Build history of the part. All positions in model axes, mm. A direction names the side the tool comes from. Round coordinates to 2 decimals unless told otherwise and drop trailing zeros. Write each loop counter-clockwise with the first axis right and the second up, starting at its lowest first coordinate (ties: lowest second). Pieces come first, ordered by that corner, then holes.
Autodesk Inventor part; units mm, degrees
ref_plane "YZ Plane" through (0, 0, 0) normal (1, 0, 0) x (0, 1, 0)
ref_plane "XZ Plane" through (0, 0, 0) normal (0, 1, 0) x (-1, 0, 0)
ref_plane "XY Plane" through (0, 0, 0) normal (0, 0, 1) x (1, 0, 0)
sketch "Sketch1" plane through (0, 0, 0) normal (0, 0, 1) x (1, 0, 0)
  line L0 (-20, 75) -> (20, 75)
  line L1 (20, 75) -> (20, -75)
  line L2 (20, -75) -> (-20, -75)
  line L3 (-20, -75) -> (-20, 75)
  line L4 (-20, 75) -> (20, -75) construction
  line L5 (20, 75) -> (-20, -75) construction
  point P0 (0, 0)
  point P1 (0, 0)
  dimension "d0" = 40
  dimension "d1" = 150
extrude "Plate1" add sketch "Sketch1" along normal blind 2
sketch "Sketch2" plane through (-20, -75, 2) normal (-1, 0, 0) x (0, -1, 0)
  line L0 (-150, 0) -> (0, 0)
  line L1 (0, 0) -> (0, 33)
  line L2 (0, 33) -> (-150, 33)
  line L3 (-150, 33) -> (-150, 0)
edge flange "Flange1" height 35 angle 90 thickness 2 bend radius 2 thickness toward (-1, 0, 0) relief tear relief width 2 relief depth 1 corner gap 2 corner form 0 edges at (-20, 0, 2) (20, 0, 2) wall of the first edge with corners at (-20, 75, 2) (-20, -75, 2) (-20, -75, 35) (-20, 75, 35)
bend "Bend1"
corner "Corner1"
sketch "Sketch3" plane through (0, 0, 0) normal (1, 0, 0) x (0, 1, 0)
  line L0 (-75, 4) -> (75, 4)
  line L1 (75, 35) -> (75, 4)
  line L2 (-75, 35) -> (75, 35)
  line L3 (-75, 4) -> (-75, 35)
  circle A0 centre (-55, 22) radius 2.5
  line L4 (-55, 22.75) -> (-55, 21.25) construction
  line L5 (-57.5, 22.75) -> (-57.5, 21.25)
  line L6 (-52.5, 21.25) -> (-52.5, 22.75)
  arc A1 (-52.5, 22.75) -> (-57.5, 22.75) centre (-55, 22.75) ccw
  arc A2 (-57.5, 21.25) -> (-52.5, 21.25) centre (-55, 21.25) ccw
  point P0 (0, 0)
  point P1 (-52.5, 22)
  point P2 (-57.5, 22)
  dimension "d13" = 5
  dimension "d14" = 13
  dimension "d15" = 20
  dimension "d29" = 1.5
extrude "Extrusion1" cut sketch "Sketch3" along normal through all both and the other way through all contours A0 | L6 A2 L5 A0 | A0 L5 A1 L6
pattern_linear "Rectangular Pattern2" count 2 spacing 100 along (0, 1, 0) of "Extrusion1"
fillet "Fillet1" radius 2 4 edges at (-21, -75, 35) (21, -75, 35) (-21, 75, 35) (21, 75, 35)
equation "\"d2\" = Thickness"
equation "\"d3\" = BendReliefWidth"
equation "\"d4\" = BendReliefDepth"
equation "\"d5\" = MinimumRemnant"
equation "\"d6\" = TransitionRadius"
equation "\"d9\" = BendRadius"
equation "\"d10\" = CornerReliefSize"
equation "\"d11\" = GapSize"
equation "\"d12\" = JacobiRadiusSize"
equation "\"BendRadius\" = Thickness"
equation "\"BendReliefWidth\" = Thickness"
equation "\"BendReliefDepth\" = 0.5 * Thickness"
equation "\"CornerReliefSize\" = 4 * Thickness"
equation "\"MinimumRemnant\" = 2 * Thickness"
equation "\"TransitionRadius\" = BendRadius"
equation "\"JacobiRadiusSize\" = BendRadius"
equation "\"GapSize\" = Thickness"
properties part number "NDM 7.44 bracket middle" material "Stainless Steel"
1) Slice it at A-A (z = 28). Write the cut outline in (x, y).
Results:
outline: (-22, -75) - (-20, -75) - (-20, 75) - (-22, 75) - close; (20, -75) - (22, -75) - (22, 75) - (20, 75) - close
2) Slice it at B-B (y = 45). Write the cut outline in (x, z).
Results:
outline: (-22, 4) arc R4 ccw to (-18, 0) - (18, 0) arc R4 ccw to (22, 4) - (22, 18.75) - (20, 18.75) - (20, 4) arc R2 cw to (18, 2) - (-18, 2) arc R2 cw to (-20, 4) - (-20, 18.75) - (-22, 18.75) - close; (-22, 25.25) - (-20, 25.25) - (-20, 35) - (-22, 35) - close; (20, 25.25) - (22, 25.25) - (22, 35) - (20, 35) - close
3) Mould opens along Y. For faces 4 (the cylindrical face through (-21.01, 45.05, 18.75)), 5 (the flat face through (0, 1, 2)), 6 (the flat face through (-2, 75, 1)) say: released by +Y, released by -Y, zero draft, split by the parting line, or undercut.
Results:
face 4: undercut
face 5: zero draft
face 6: released by +Y
4) Slice it at D-D (x = 6.5). Write the cut outline in (y, z).
Results:
outline: (-75, 0) - (75, 0) - (75, 2) - (-75, 2) - close
5) Slice it at C-C (y = 9.5). Write the cut outline in (x, z).
Results:
outline: (-22, 4) arc R4 ccw to (-18, 0) - (18, 0) arc R4 ccw to (22, 4) - (22, 35) - (20, 35) - (20, 4) arc R2 cw to (18, 2) - (-18, 2) arc R2 cw to (-20, 4) - (-20, 35) - (-22, 35) - close
6) Which spindle directions (+Z, -Z, +X, -X, +Y, -Y) get a long thin tool onto all of the face, cutting with end or side? Do faces 1 (the cylindrical face through (-21.01, 44.95, 25.25)), 2 (the flat face through (0, 1, 0)), 3 (the flat face through (-20, -1, 19)). Say none if no direction does.
Results:
face 1: +X, -X
face 2: -Z, +X, -X, +Y, -Y
face 3: +Z, +Y, -Y
7) Pin check, flat tips, straight feed: pin 1 Ø4 at (x, y) = (7.5, 27) entering from +Z; pin 2 Ø12 at (x, z) = (-10, 28.5) entering from -Y; pin 3 Ø3 at (x, y) = (14.5, 52.5) entering from -Z. Stop position of each tip, or through.
Results:
pin 1: stops at z = 2
pin 2: passes through
pin 3: stops at z = 0
8) Wall check: L1, parallel to X at y = 37, z = 19; L2, parallel to Z at x = -13.5, y = 63; L3, parallel to Z at x = 18.5, y = -4. Give the ranges that are in metal, low to high.
Results:
L1: x = -22 to -20, 20 to 22
L2: z = 0 to 2
L3: z = 0.03 to 2.06
